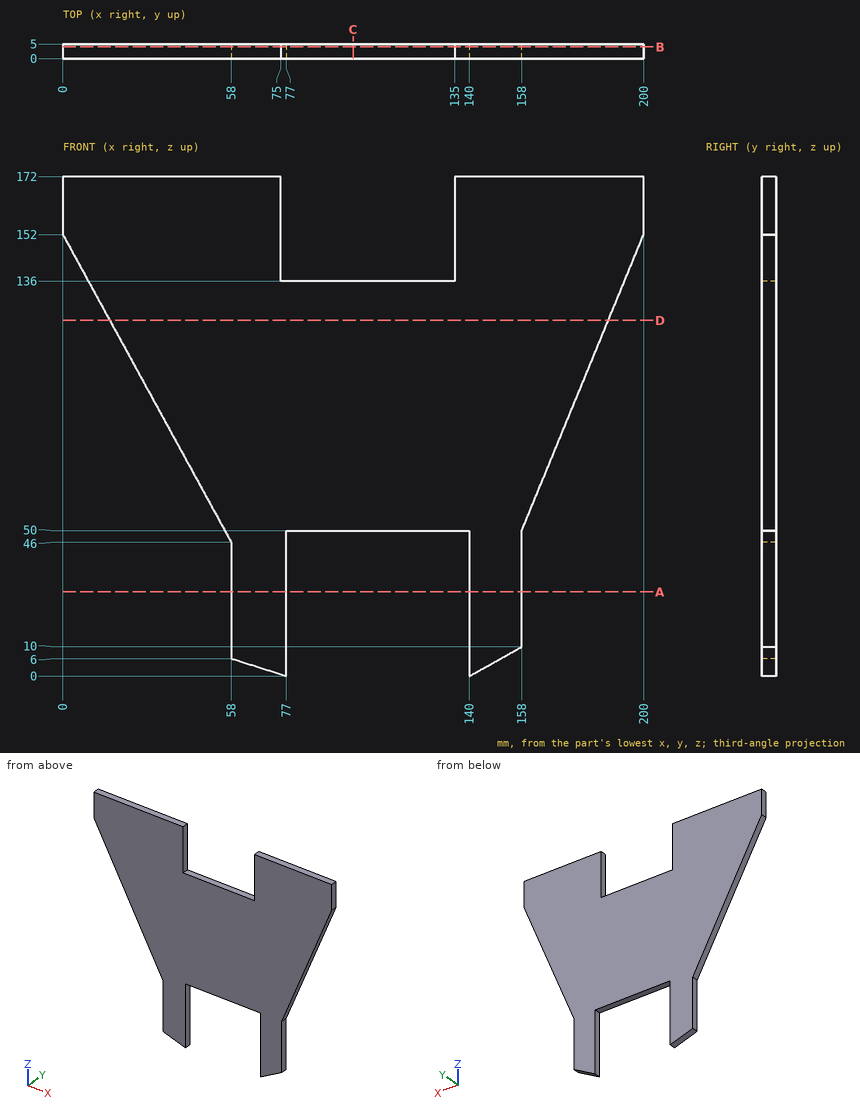
Verification items for this drawing (mm, ordinates from the low corner). Give positions to 0.01 mm unless a question says otherwise; leave off trailing zeros. Write each loop counter-clockwise with the first axis right and the second up, starting at its lowest first coordinate (ties: lowest second). Pieces come first, ordered by that corner, then holes.
1) Section check A-A, the plane z = 29. Record the boundary of the cut face in (x, y).
2) Gauge pin test, flat ends, axial feed: pin 1 (3 mm diameter, centred on x = 79, y = 4, fed in from -Z); pin 2 (1 mm diameter, centred on x = 68, y = 3.5, fed in from -Z); pin 3 (2.5 mm diameter, centred on x = 91, y = 2.5, fed in from +Z). Record the tip position at first contact, or that the pin passes through.
3) Section check D-D, the plane z = 122.5. Record the boundary of the cut face in (x, y).
4) Material ranges on L1, parallel to X at y = 2.25, z = 161.5; L2, parallel to X at y = 2.9, z = 43.5; L3, parallel to Z at x = 100, y = 3.9, recorded low to high.
5) Section check B-B, the plane y = 4. Record the boundary of the cut face in (x, z).
6) Section check C-C, the plane x = 100. Record the boundary of the cut face in (y, z), and give its area (3 significant figures).
Computed:
1. outline: (58, 0) - (77, 0) - (77, 5) - (58, 5) - close; (140, 0) - (158, 0) - (158, 5) - (140, 5) - close
2. pin 1: stops at z = 50
2. pin 2: stops at z = 2.68
2. pin 3: stops at z = 136
3. outline: (16.14, 0) - (187.85, 0) - (187.85, 5) - (16.14, 5) - close
4. L1: x = 0 to 75, 135 to 200
4. L2: x = 58 to 77, 140 to 158
4. L3: z = 50 to 136
5. outline: (0, 152) - (58, 46) - (58, 6) - (77, 0) - (77, 50) - (140, 50) - (140, 0) - (158, 10) - (158, 50) - (200, 152) - (200, 172) - (135, 172) - (135, 136) - (75, 136) - (75, 172) - (0, 172) - close
6. outline: (0, 50) - (5, 50) - (5, 136) - (0, 136) - close
6. area: 430 mm2
